from build123d import *

# Parameters (mm, degrees)
CROQUIS1_R              = 1.5
SALIENTE_EXTRUIR1_DEPTH = 2


with BuildPart() as part:
    # Croquis1 → Saliente-Extruir1 (new body)
    with BuildSketch(Plane(origin=(0, 0, 0), x_dir=(1, 0, 0), z_dir=(0, 1, 0))):
        with BuildLine():
            Line((-30, 79.023809524), (-30, 0))
            Line((-30, 0), (-30, -63.476190476))
            Line((-30, -63.476190476), (-13.983050847, -63.476190476))
            Line((-13.983050847, -63.476190476), (0, 46.523809524))
            Line((0, 46.523809524), (-15, 76.523809524))
            Line((-15, 76.523809524), (-15, 79.023809524))
            ThreePointArc((-15, 79.023809524), (-22.5, 86.523809524), (-30, 79.023809524))
        make_face()
        with Locations(Location((-22.5, 79.023809524, 0), (0, 0, 270))):
            Circle(CROQUIS1_R, mode=Mode.SUBTRACT)
    extrude(amount=SALIENTE_EXTRUIR1_DEPTH)


solid = part.part
Build history of the part. All positions in model axes, mm. Give positions to 0.01 mm unless a question says otherwise; leave off trailing zeros. Order: outer loops, then holes, each group sorted by start corner. A loop starts at its lowest first (then second) coordinate and runs counter-clockwise, first axis right, second up. Notation, with made-up numbers: M 31.5,72 L 56.5,72 A10 cw 56.5,85 Z; hole C 19.5,37.5 d5. An arc over 180 degrees is marked long. Use one line per item in the form item = value.
1) Drop a flat-ended pin along its axis: pin 1 (2 mm diameter, centred on x = -18, z = -0.5, fed in from -Y). Give the stop position or say it passes through.
Calculated:
pin_1 = 0
2) Saw through at D-D (z = 16). Give the cut face in (x, y), plus the area to 3 significant figures.
Calculated:
outline = M -30,0 L -7.95,0 L -7.95,2 L -30,2 Z
area = 44.1 mm2
3) Two-plate mould, pull along X, no slides. Class faces 1 (the face through (-19, 2, -13)), 2 (the face through (-22.434, 0.986, -80.522)), 3 (the face through (-7.09, 0.99, 9.25)), 4 (the face through (-22.335, 0.986, -86.522)): released by +X, released by -X, zero draft, split by the parting line, or undercut.
Calculated:
face_1 = zero draft
face_2 = undercut
face_3 = released by +X
face_4 = split by the parting line
4) Saw through at C-C (x = -4.75). Give the cut face in (y, z).
Calculated:
outline = M 0,-56.02 L 2,-56.02 L 2,-9.16 L 0,-9.16 Z
5) Saw through at B-B (x = -22.5). Give the cut face in (y, z).
Calculated:
outline = M 0,-86.52 L 2,-86.52 L 2,-80.52 L 0,-80.52 Z; M 0,-77.52 L 2,-77.52 L 2,63.48 L 0,63.48 Z
6) Probe probe 1 along Z at (x, y) = (-22.25, 1.9); probe 2 along X at (y, z) = (0.1, -78.5); probe 3 along Z at (x, y) = (-23.5, 1.1). List the from-to ranges inside material, lowest first.
Calculated:
probe_1 = -86.52 to -80.5, -77.54 to 63.48
probe_2 = -30 to -23.91, -21.09 to -15
probe_3 = -86.46 to -80.14, -77.91 to 63.48
7) Saw through at A-A (y = 1.6). Give the cut face in (x, z), plus the area to 3 significant figures.
Calculated:
outline = M -30,-79.02 A7.5 ccw -15,-79.02 L -15,-76.52 L 0,-46.52 L -13.98,63.48 L -30,63.48 Z; hole C -22.5,-79.02 d3
area = 3,320 mm2
